from build123d import *

# Parameters (mm, degrees)
SKETCH2_R               = 2.5
CUT_EXTRUDE3_DEPTH      = 92.175654645
CUT_EXTRUDE6_DEPTH      = 93.352585237
CUT_EXTRUDE6_DEPTH_BACK = 93.352585237
SKETCH6_R               = 2.5


with BuildPart() as part:
    # Sketch1 → Revolve1 (revolve)
    with BuildSketch(Plane.XY, mode=Mode.PRIVATE) as revolve1_sk:
        Polygon((-42, -29), (-42, -4), (-62, -4), (-62, 0), (-38, 0), (-38, -29), align=None)
    revolve(revolve1_sk.sketch.rotate(Axis((0, -100.5, 0), (0, 1, 0)), 270), axis=Axis((0, -100.5, 0), (0, 1, 0)))

    # Sketch2 → Cut-Extrude3 (cut, through all)
    with BuildSketch(Plane.XZ.offset(4)):
        with Locations(Location((55, 0, 0), (0, 0, 270))):
            Circle(SKETCH2_R)
        with Locations(Location((-55, 0, 0), (0, 0, 270))):
            Circle(SKETCH2_R)
        with Locations(Location((0, 55, 0), (0, 0, 270))):
            Circle(SKETCH2_R)
        with Locations(Location((0, -55, 0), (0, 0, 270))):
            Circle(SKETCH2_R)
    extrude(amount=-CUT_EXTRUDE3_DEPTH, mode=Mode.SUBTRACT)

    # Sketch6 → Cut-Extrude6 (cut, two sides: drawn at the far end of the back side and taken through both)
    with BuildSketch(Plane.XY.offset(-CUT_EXTRUDE6_DEPTH_BACK)):
        with Locations((0, -19)):
            Circle(SKETCH6_R)
    extrude(amount=CUT_EXTRUDE6_DEPTH + CUT_EXTRUDE6_DEPTH_BACK, mode=Mode.SUBTRACT)


solid = part.part
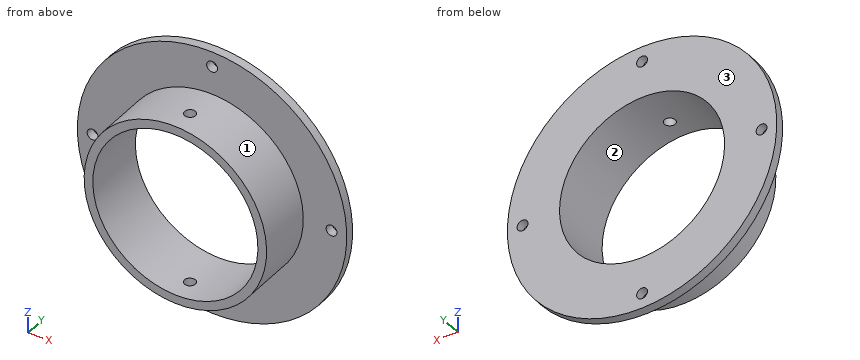
Input: part model. Units: mm. Frame: model coordinates. Face numbers are marked on the shaded views. Round coordinates to 2 decimals unless told otherwise and drop trailing zeros. Order: outer loops, then holes, each group sorted by start corner. A loop starts at its lowest first (then second) coordinate and runs counter-clockwise, first axis right, second up.
1. Material intervals for line 1 (X direction, y = -15.25, z = 0); line 2 (Y direction, x = 0, z = 39); line 3 (Y direction, x = 46, z = -10), sorted ascending.
The answers:
line 1: x = -42 to -38, 38 to 42
line 2: y = -29 to -21.5, -16.5 to 0
line 3: y = -4 to 0
2. Mould query, pull axis X, two halves, no side actions, for the marked faces 1, 2 and 3. Classes: released by +X, released by -X, zero draft, split by the parting line, or undercut.
The answers:
face 1: split by the parting line
face 2: undercut
face 3: zero draft
3. Pin query (flat end, axial travel): P1, Ø4.5, axis at x = 0, y = -19, coming from the +Z side; P2, Ø6, axis at y = -19.5, z = -22, coming from the +X side; P3, Ø8, axis at y = -12, z = 19.5, coming from the +X side; P4, Ø1, axis at y = -19.5, z = -30, coming from the +X side. Return the tip coordinate at first contact, or that it passes through.
The answers:
P1: passes through
P2: stops at x = 37.46
P3: stops at x = 39.04
P4: stops at x = 29.9
4. Cut plane D-D, the plane z = 14. Output: boundary loops of the cut face in (x, y).
The answers:
outline: (-60.4, -4) - (-39.6, -4) - (-39.6, -29) - (-35.33, -29) - (-35.33, 0) - (-60.4, 0) - close; (35.33, -29) - (39.6, -29) - (39.6, -4) - (60.4, -4) - (60.4, 0) - (35.33, 0) - close
5. Cut plane B-B, the plane x = -55. Output: boundary loops of the cut face in (y, z), then the cut area to 3 significant figures.
The answers:
outline: (-4, -28.62) - (0, -28.62) - (0, -2.5) - (-4, -2.5) - close; (-4, 2.5) - (0, 2.5) - (0, 28.62) - (-4, 28.62) - close
area: 209 mm2
6. Cut plane C-C, the plane x = 0. Output: boundary loops of the cut face in (y, z).
The answers:
outline: (-29, -42) - (-21.5, -42) - (-21.5, -38) - (-29, -38) - close; (-29, 38) - (-21.5, 38) - (-21.5, 42) - (-29, 42) - close; (-16.5, -42) - (-4, -42) - (-4, -52.5) - (0, -52.5) - (0, -38) - (-16.5, -38) - close; (-16.5, 38) - (0, 38) - (0, 52.5) - (-4, 52.5) - (-4, 42) - (-16.5, 42) - close; (-4, -62) - (0, -62) - (0, -57.5) - (-4, -57.5) - close; (-4, 57.5) - (0, 57.5) - (0, 62) - (-4, 62) - close
7. Cut plane A-A, the plane z = 0. Output: boundary loops of the cut face in (x, y), then the cut area to 3 significant figures.
The answers:
outline: (-62, -4) - (-57.5, -4) - (-57.5, 0) - (-62, 0) - close; (-52.5, -4) - (-42, -4) - (-42, -29) - (-38, -29) - (-38, 0) - (-52.5, 0) - close; (38, -29) - (42, -29) - (42, -4) - (52.5, -4) - (52.5, 0) - (38, 0) - close; (57.5, -4) - (62, -4) - (62, 0) - (57.5, 0) - close
area: 352 mm2
